from build123d import *

# Parameters (mm, degrees)
SKETCH1_R           = 12.5
BOSS_EXTRUDE1_DEPTH = 1.5
SKETCH2_W           = 9.8
SKETCH2_H           = 9.8
BOSS_EXTRUDE2_DEPTH = 4.25
SKETCH3_R           = 12.5
BOSS_EXTRUDE3_DEPTH = 47.5
SKETCH4_R           = 12.5
BOSS_EXTRUDE4_DEPTH = 3
SKETCH5_R           = 12.5
SKETCH5_R_2         = 11.5
BOSS_EXTRUDE5_DEPTH = 6.5


with BuildPart() as part:
    # Sketch1 → Boss-Extrude1 (new, symmetric)
    with BuildSketch(Plane(origin=(0, 0, 0), x_dir=(1, 0, 0), z_dir=(0, 1, 0))):
        with Locations(Location((0, 0, 0), (0, 0, 270))):
            Circle(SKETCH1_R)
    boss_extrude1 = extrude(amount=BOSS_EXTRUDE1_DEPTH, both=True)

    # Sketch2 → Boss-Extrude2 (add)
    with BuildSketch(Plane(origin=(0, 1.5, 0), x_dir=(1, 0, 0), z_dir=(0, 1, 0))):
        Rectangle(SKETCH2_W, SKETCH2_H)
    extrude(amount=BOSS_EXTRUDE2_DEPTH)

    # Mirror1: Boss-Extrude1 across plane
    add(boss_extrude1.mirror(Plane.ZX.offset(3.625)))

    # Sketch3 → Boss-Extrude3 (add)
    with BuildSketch(Plane(origin=(0, 8.75, 0), x_dir=(1, 0, 0), z_dir=(0, 1, 0))):
        with Locations(Location((0, 0, 0), (0, 0, 270))):
            Circle(SKETCH3_R)
    extrude(amount=BOSS_EXTRUDE3_DEPTH)

    # Sketch4 → Boss-Extrude4 (add)
    with BuildSketch(Plane(origin=(0, 56.25, 0), x_dir=(1, 0, 0), z_dir=(0, 1, 0))):
        with Locations(Location((0, 0, 0), (0, 0, 270))):
            Circle(SKETCH4_R)
    extrude(amount=BOSS_EXTRUDE4_DEPTH)

    # Sketch5 → Boss-Extrude5 (add)
    with BuildSketch(Plane(origin=(0, 59.25, 0), x_dir=(1, 0, 0), z_dir=(0, 1, 0))):
        with Locations(Location((0, 0, 0), (0, 0, 270))):
            Circle(SKETCH5_R)
        with Locations(Location((0, 0, 0), (0, 0, 90))):
            Circle(SKETCH5_R_2, mode=Mode.SUBTRACT)
    extrude(amount=BOSS_EXTRUDE5_DEPTH)


solid = part.part
Could you check a few things on this model? Use its own coordinates, in mm. A direction names the side the tool comes from. Coordinates: 2 decimals unless noted, no trailing zeros. Loops run counter-clockwise (first coordinate to the right, second up) from the corner with the lowest first, then second, coordinate; pieces in that order, holes last.
1. Imagine slicing it at C-C (x = 0). Please give me the cut outline in (y, z), and give its area (3 significant figures).
2. Imagine slicing it at B-B (z = 0). Please give me the cut outline in (x, y), and give its area (3 significant figures).
3. We'd pull the mould along Z, two halves only. Please class faces 1 (the face through (0, 59.25, 0)), 2 (the face through (-5.4, 1.5, -0.2)), 3 (the face through (3.755, 35.33, 11.923)): released by +Z, released by -Z, zero draft, split by the parting line, or undercut.
4. I need wall thicknesses on L1, parallel to Y at x = -0.25, z = 8.25; L2, parallel to X at y = 61.5, z = 0; L3, parallel to Y at x = 2, z = 1.5. Which ranges of each line are inside material? Lowest first, please.
5. For faces 4 (the face through (-9.7, 62.45, -6.18)), 5 (the face through (-4.9, 4, 0)), 6 (the face through (-5.4, 5.75, -0.2)), which set-ups out of +Z, -Z, +X, -X, +Y, -Y let a thin tool reach every point of the face, with its end or its side?
6. For P1, Ø1.3, axis at x = -2, y = 3, coming from the +Z side; P2, Ø1.5, axis at x = -0.5, z = -4, coming from the +Y side; P3, Ø2, axis at y = 4.5, z = 0.5, coming from the -X side, each with a flat end and sliding along its axis, tell me the tip position at first contact or that it passes through.
7. Imagine slicing it at A-A (z = 10). Please give me the cut outline in (x, y).
8. Imagine slicing it at D-D (y = 16.5). Please give me the cut outline in (x, z), and give its area (3 significant figures).
Computed values:
1. outline: (-1.5, -12.5) - (1.5, -12.5) - (1.5, -4.9) - (5.75, -4.9) - (5.75, -12.5) - (65.75, -12.5) - (65.75, -11.5) - (59.25, -11.5) - (59.25, 11.5) - (65.75, 11.5) - (65.75, 12.5) - (5.75, 12.5) - (5.75, 4.9) - (1.5, 4.9) - (1.5, 12.5) - (-1.5, 12.5) - close
1. area: 1,470 mm2
2. outline: (-12.5, -1.5) - (12.5, -1.5) - (12.5, 1.5) - (4.9, 1.5) - (4.9, 5.75) - (12.5, 5.75) - (12.5, 65.75) - (11.5, 65.75) - (11.5, 59.25) - (-11.5, 59.25) - (-11.5, 65.75) - (-12.5, 65.75) - (-12.5, 5.75) - (-4.9, 5.75) - (-4.9, 1.5) - (-12.5, 1.5) - close
2. area: 1,470 mm2
3. face 1: undercut
3. face 2: zero draft
3. face 3: split by the parting line
4. L1: y = -1.5 to 1.5, 5.75 to 59.25
4. L2: x = -12.5 to -11.5, 11.5 to 12.5
4. L3: y = -1.5 to 59.25
5. face 4: +Y
5. face 5: +Z, -Z, -X
5. face 6: none
6. P1: stops at z = 4.9
6. P2: stops at y = 59.25
6. P3: stops at x = -4.9
7. outline: (-7.5, -1.5) - (7.5, -1.5) - (7.5, 1.5) - (-7.5, 1.5) - close; (-7.5, 5.75) - (7.5, 5.75) - (7.5, 65.75) - (5.68, 65.75) - (5.68, 59.25) - (-5.68, 59.25) - (-5.68, 65.75) - (-7.5, 65.75) - close
8. outline: circle Ø25 at (0, 0)
8. area: 491 mm2
